Print and shaded views of the part. All mm, measured from the part's lowest x, y and z. Round coordinates to 2 decimals unless told otherwise and drop trailing zeros. Write each loop counter-clockwise with the first axis right and the second up, starting at its lowest first coordinate (ties: lowest second). Pieces come first, ordered by that corner, then holes. Notation, with made-up numbers: (71, -28) - (123, -28) arc R7 ccw to (123, -18) - close; hole circle Ø3 at (1, -4.5). An arc over 180 degrees is marked (long way). Answer as a JSON object with one key per item and string values. Group by question number.
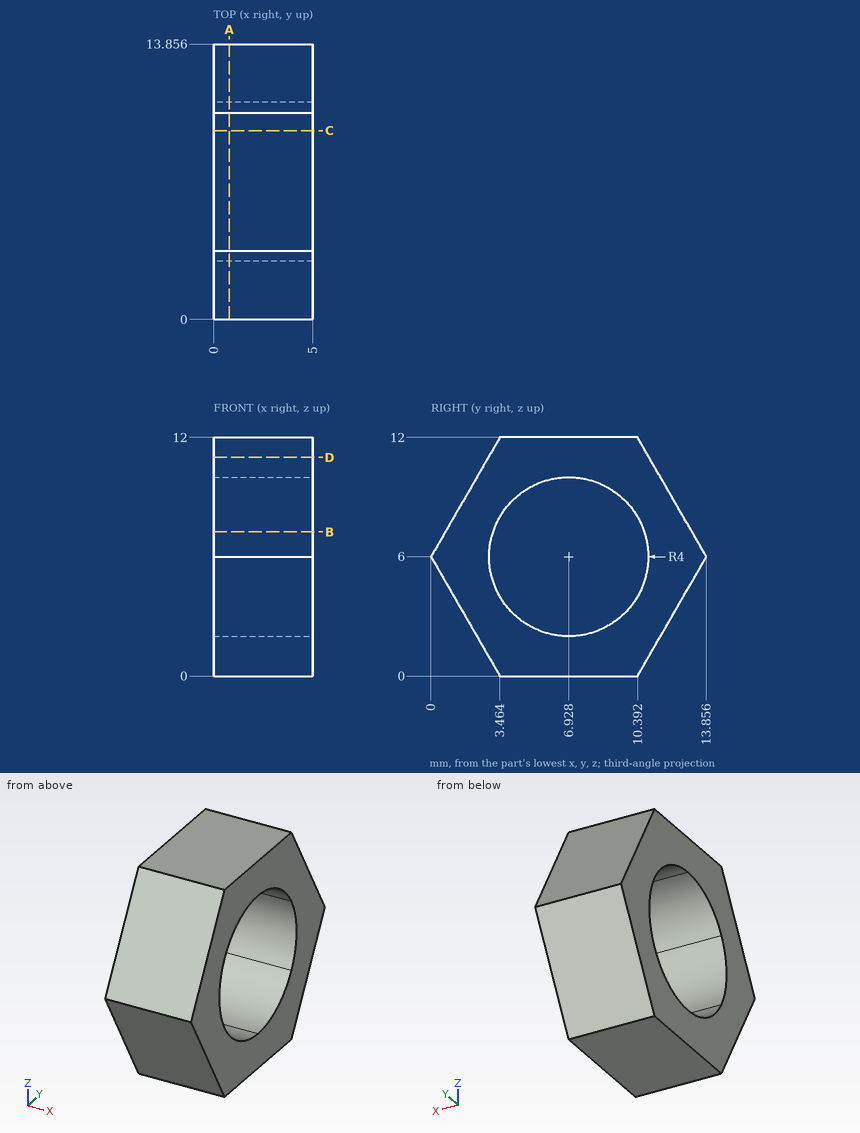
(1) Slice it at A-A (x = 0.8). Write the cut outline in (y, z).
(2) Slice it at D-D (z = 11). Write the cut outline in (x, y).
(3) Drill centre lines: line 1 (Y direction, x = 1.3, z = 5) (1 decimal); line 2 (Z direction, x = 1.9, y = 10); line 3 (Z direction, x = 2.3, y = 10.5) (1 decimal). Where is each one in solid material? Low to high. Write a range as from..to.
(4) Slice it at B-B (z = 7.25). Write the cut outline in (x, y) (1 decimal).
(5) Slice it at C-C (y = 9.5). Write the cut outline in (x, z).
(6) Flat gauge pins, fed straight in: pin 1 (1.5 mm diameter, centred on y = 5, z = 4, fed in from +X); pin 2 (2 mm diameter, centred on x = 3.5, z = 2, fed in from -Y); pin 3 (1 mm diameter, centred on y = 4.5, z = 9, fed in from -X). Where does each tip first touch, or does it go through?
Answer:
{
 "1": {"outline": "(0, 6) - (3.46, 0) - (10.39, 0) - (13.86, 6) - (10.39, 12) - (3.46, 12) - close; hole circle Ø8 at (6.93, 6)"},
 "2": {"outline": "(0, 2.89) - (5, 2.89) - (5, 10.97) - (0, 10.97) - close"},
 "3": {"line 1": "0.6..3.1, 10.8..13.3", "line 2": "0..3.44, 8.56..12", "line 3": "0.2..4.2, 7.8..11.8"},
 "4": {"outline": "(0, 0.7) - (5, 0.7) - (5, 3.1) - (0, 3.1) - close; (0, 10.7) - (5, 10.7) - (5, 13.1) - (0, 13.1) - close"},
 "5": {"outline": "(0, 0) - (5, 0) - (5, 2.94) - (0, 2.94) - close; (0, 9.06) - (5, 9.06) - (5, 12) - (0, 12) - close"},
 "6": {"pin 1": "through", "pin 2": "y = 1.73", "pin 3": "x = 0"}
}
